from build123d import *

# Parameters (mm, degrees)
F0_W      = 355
F0_H      = 215
F1_DEPTH  = 1.1
F2_W      = 38
F2_H      = 22
F2_W_2    = 34
F3_DEPTH  = 0.95
F4_W      = 22
F4_H      = 157
F5_DEPTH  = 0.95
F6_W      = 22
F6_H      = 179
F7_DEPTH  = 0.95
F8_W      = 64
F8_H      = 179
F9_DEPTH  = 0.95
F11_DEPTH = 0.95
F13_DEPTH = 0.95
F15_DEPTH = 0.95
F17_DEPTH = 0.95


with BuildPart() as f1:
    # F0 (on Top) → F1 (new body)
    with BuildSketch(Plane.XY):
        Rectangle(F0_W, F0_H)
    extrude(amount=F1_DEPTH)

    # F2 (on face) → F3 (join)
    with BuildSketch(Plane.XY.offset(1.1)):
        Polygon((-88.5, 89.5), (-110.5, 89.5), (-110.5, -89.5), (-88.5, -89.5), (-88.5, -67.5), (-88.5, -4.988748), (-88.5, 17.011252), (-88.5, 67.5), align=None)
        with Locations((-69.5, 78.5)):
            Rectangle(F2_W, F2_H)
        with Locations((-69.5, -78.5)):
            Rectangle(F2_W, F2_H)
        with Locations((-71.5, 6.011252)):
            Rectangle(F2_W_2, F2_H)
    extrude(amount=F3_DEPTH)

    # F4 (on face) → F5 (join)
    with BuildSketch(Plane.XY.offset(1.1)):
        Polygon((130.5, 89.5), (68.5, 89.5), (68.5, 67.5), (88.5, 67.5), (110.5, 67.5), (130.5, 67.5), align=None)
        with Locations((99.5, -11)):
            Rectangle(F4_W, F4_H)
    extrude(amount=F5_DEPTH)

    # F6 (on face) → F7 (join)
    with BuildSketch(Plane.XY.offset(1.1)):
        with Locations((46.5, 0)):
            Rectangle(F6_W, F6_H)
    extrude(amount=F7_DEPTH)

    # F8 (on face) → F9 (join)
    with BuildSketch(Plane.XY.offset(1.1)):
        with Locations((-7.5, -1)):
            Rectangle(F8_W, F8_H)
    extrude(amount=F9_DEPTH)

    # F10 (on face) → F11 (cut)
    with BuildSketch(Plane.XY.offset(2.05)):
        Polygon((-15.5, -1), (-39.5, 88.5), (-39.5, -90.5), align=None)
    extrude(amount=-F11_DEPTH, mode=Mode.SUBTRACT)

    # F12 (on face) → F13 (cut)
    with BuildSketch(Plane.XY.offset(2.05)):
        Polygon((24.5, -90.5), (24.5, 88.5), (0.5, 0), align=None)
    extrude(amount=-F13_DEPTH, mode=Mode.SUBTRACT)

    # F14 (on face) → F15 (cut)
    with BuildSketch(Plane.XY.offset(2.05)):
        Polygon((-7.5, -43.495346), (-19.85, -90.5), (4.85, -90.5), align=None)
    extrude(amount=-F15_DEPTH, mode=Mode.SUBTRACT)

    # F16 (on face) → F17 (cut)
    with BuildSketch(Plane.XY.offset(2.05)):
        Polygon((4.85, 88.5), (-19.85, 88.5), (-7.5, 41.495346), align=None)
    extrude(amount=-F17_DEPTH, mode=Mode.SUBTRACT)


solid = f1.part
Model file for the job. Use its own axes, mm. A direction names the side the tool comes from. Round coordinates to 2 decimals unless told otherwise and drop trailing zeros. Loops run counter-clockwise (first coordinate to the right, second up) from the corner with the lowest first, then second, coordinate; pieces in that order, holes last. Notation, with made-up numbers: M -32,42.5 L 9,42.5 A21 cw 9,75.5 Z; hole C 50,-37 d11. An arc over 180 degrees is marked long. One line per question, with ' | ' between items.
1) Mould opens along X. For faces 6 (the flat face through (-42, 2, 1.1)), 7 (the flat face through (-13.761, 65.327, 1.582)), 8 (the flat face through (46, 1, 2.05)) say: +X half, -X half, draft (parallel to the pull), parting line (faces both ways), or undercut.
Solved:
face 6: undercut | face 7: undercut | face 8: draft
2) Band-saw the part on A-A (x = 53). Give the cut face in (y, z).
Solved:
outline: M -107.5,0 L 107.5,0 L 107.5,1.1 L 89.5,1.1 L 89.5,2.05 L -89.5,2.05 L -89.5,1.1 L -107.5,1.1 Z
3) 3-axis set-ups, long thin cutter, end or side, ignore diameter. For faces 1 (the flat face through (-2, 2, 0)), 2 (the flat face through (-13.59, -66.67, 1.58)), 3 (the flat face through (-1.41, 64.67, 1.58)), 4 (the flat face through (-8, 0, 2.05)), 5 (the flat face through (-27.33, 43.12, 1.58)): which of +Z, -Z, +X, -X, +Y, -Y reach the whole face in a straight line?
Solved:
face 1: -Z, +X, -X, +Y, -Y | face 2: +Z, -Y | face 3: +Z, +Y | face 4: +Z, +X, -X, +Y, -Y | face 5: +Z
4) Flat gauge pins, fed straight in: pin 1 (0.5 mm diameter, centred on x = 43.5, z = 2, fed in from +Y); pin 2 (1 mm diameter, centred on x = -114, y = -43, fed in from +Z); pin 3 (0.5 mm diameter, centred on x = -28.5, z = 1.5, fed in from +Y). Where does each tip first touch, or does it go through?
Solved:
pin 1: stops at y = 89.5 | pin 2: stops at z = 1.1 | pin 3: stops at y = 88.5
5) Band-saw the part on B-B (z = 1.6). Give the number of separate pieces and of enclosed holes in the cut face, then the cut area to 3 significant figures.
Solved:
separate pieces: 4 | enclosed holes: 0 | area: 21,100 mm²
6) Band-saw the part on C-C (y = -27). Give the cut face in (x, z).
Solved:
outline: M -177.5,0 L 177.5,0 L 177.5,1.1 L 110.5,1.1 L 110.5,2.05 L 88.5,2.05 L 88.5,1.1 L 57.5,1.1 L 57.5,2.05 L 35.5,2.05 L 35.5,1.1 L 7.66,1.1 L 7.66,2.05 L -22.47,2.05 L -22.47,1.1 L -88.5,1.1 L -88.5,2.05 L -110.5,2.05 L -110.5,1.1 L -177.5,1.1 Z
7) Band-saw the part on D-D (x = 143). Give the cut face in (y, z), then the cut area to 4 significant figures.
Solved:
outline: M -107.5,0 L 107.5,0 L 107.5,1.1 L -107.5,1.1 Z | area: 236.5 mm²
8) Drill centre lines: line 1 along X through (y, z) = (-54, 1.45); line 2 along X through (y, z) = (68.5, 1.6); line 3 along X through (y, z) = (6, 1.6). Where is each one in solid material? Low to high.
Solved:
line 1: x = -110.5 to -88.5, -29.71 to -10.26, -4.74 to 14.82, 35.5 to 57.5, 88.5 to 110.5 | line 2: x = -110.5 to -50.5, -34.14 to -14.6, -0.4 to 19.08, 35.5 to 57.5, 68.5 to 130.5 | line 3: x = -110.5 to -54.5, -17.38 to 2.13, 35.5 to 57.5, 88.5 to 110.5
